Geometry check sheet. Reference: drawing and pictorial views, mm from the part's lowest x, y, z. A direction names the side the tool comes from. Give positions to 0.01 mm unless a question says otherwise; leave off trailing zeros. Write each loop counter-clockwise with the first axis right and the second up, starting at its lowest first coordinate (ties: lowest second). Pieces come first, ordered by that corner, then holes. Notation, with made-up numbers: (-33, 51) - (-26, 51) arc R10 cw to (-26, 66) - close; hole circle Ø1 at (-24.5, -18). An arc over 180 degrees is marked (long way). Write item = value, one per line. Start each with the question number.
(1) Access from +Z, -Z, +X, -X, +Y, -Y to the whole of each face (thin tool, end or side, straight path). Record for the marked faces 4 and 5.
(2) Draft check along Y on the marked faces 1, 2 and 3. Enter one of: pulls with the +Y half, pulls with the -Y half, needs draft (parallel to the pull), parting line crosses it, or undercut.
(3) Depth check by flat-ended pin: pin 1 Ø2 at (x, z) = (26.5, 38.5) entering from -Y. Enter the tip coordinate at first touch or a pass-through.
(4) Thickness scan on L1, parallel to Z at x = 38.1, y = 24.4; L2, parallel to X at y = 2.25, z = 86.5; L3, parallel to Y at x = 50, z = 95. Record the ranges inside material, lowest first.
(5) Section check C-C, the plane z = 95.25. Enter the section's corners in (x, y), plus the area to 3 significant figures.
(6) Section check A-A, the plane y = 19.75. Enter the section's corners in (x, z).
(7) Section check B-B, the plane x = 20. Enter the section's corners in (y, z).
(8) Section check D-D, the plane z = 33. Enter the section's corners in (x, y).
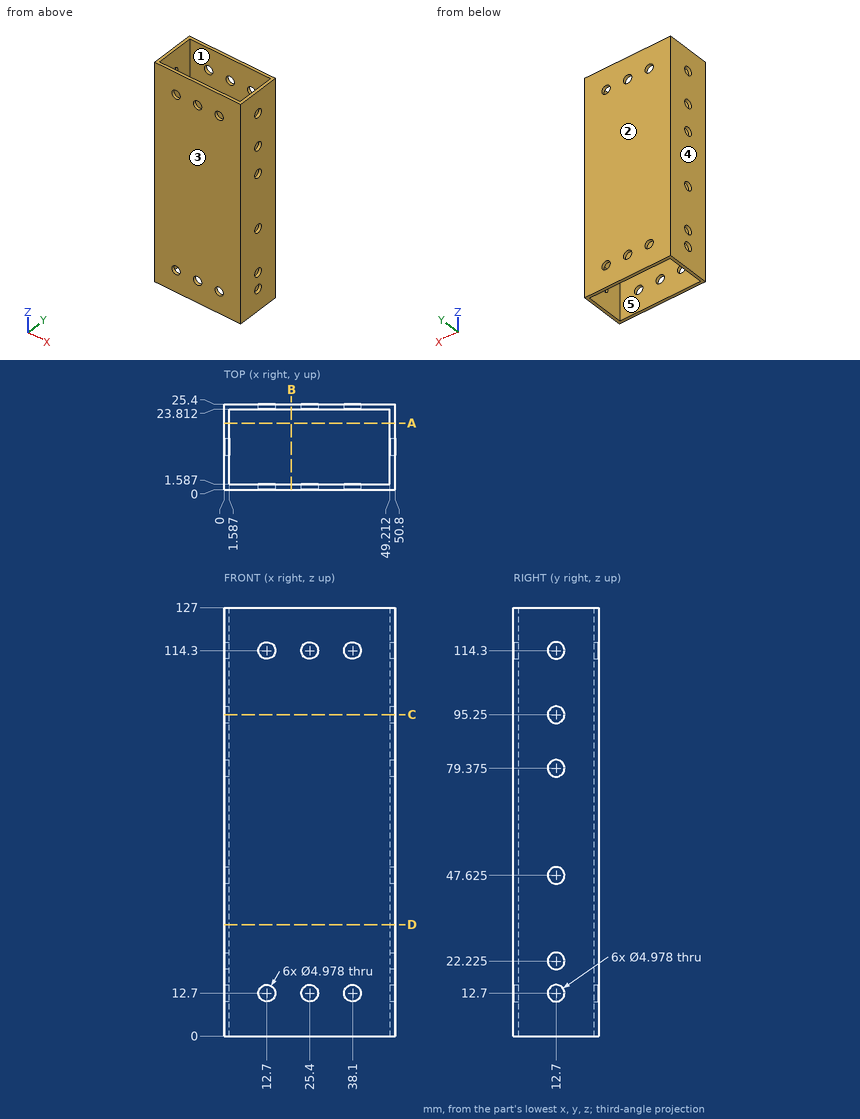
Model answer:
q1.face_4 = +Z, -Z, -X, +Y, -Y
q1.face_5 = +Z, -Z
q2.face_1 = undercut
q2.face_2 = pulls with the +Y half
q2.face_3 = pulls with the -Y half
q3.pin_1 = 0
q4.L1 = 0 to 10.21, 15.19 to 111.81, 116.79 to 127
q4.L2 = 0 to 1.59, 49.21 to 50.8
q4.L3 = 0 to 10.22, 15.18 to 25.4
q5.outline = (0, 0) - (50.8, 0) - (50.8, 10.21) - (49.21, 10.21) - (49.21, 1.59) - (1.59, 1.59) - (1.59, 10.21) - (0, 10.21) - close; (0, 15.19) - (1.59, 15.19) - (1.59, 23.81) - (49.21, 23.81) - (49.21, 15.19) - (50.8, 15.19) - (50.8, 25.4) - (0, 25.4) - close
q5.area = 216 mm²
q6.outline = (0, 0) - (1.59, 0) - (1.59, 127) - (0, 127) - close; (49.21, 0) - (50.8, 0) - (50.8, 127) - (49.21, 127) - close
q7.outline = (0, 0) - (1.59, 0) - (1.59, 127) - (0, 127) - close; (23.81, 0) - (25.4, 0) - (25.4, 127) - (23.81, 127) - close
q8.outline = (0, 0) - (50.8, 0) - (50.8, 25.4) - (0, 25.4) - close; hole (1.59, 1.59) - (49.21, 1.59) - (49.21, 23.81) - (1.59, 23.81) - close
